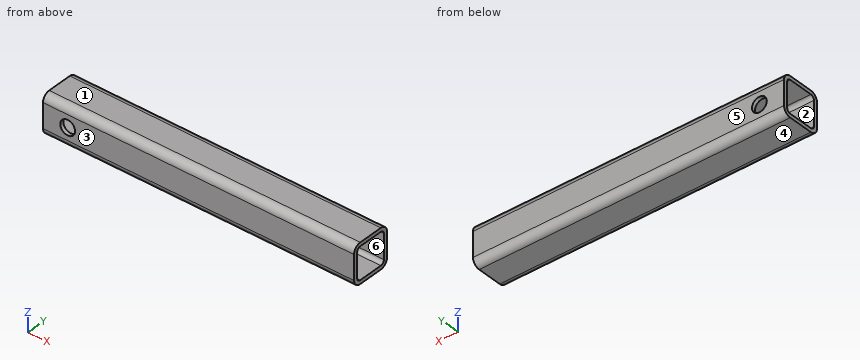
from build123d import *

# Parameters (mm, degrees)
TUBE_SQUARE_TS2X2X0_1875_1_DEPTH = 400
SKETCH12_R                       = 9.525
CUT_EXTRUDE1_DEPTH               = 405.012128531


with BuildPart() as part:
    # Sketch11 → Tube square TS2X2X0.1875(1) (new body)
    with BuildSketch(Plane.YZ):
        with BuildLine():
            Line((-15.875, -25.4), (15.875, -25.4))
            ThreePointArc((15.875, -25.4), (22.610192091, -22.610192091), (25.4, -15.875))
            Line((25.4, -15.875), (25.4, 15.875))
            ThreePointArc((25.4, 15.875), (22.610192091, 22.610192091), (15.875, 25.4))
            Line((15.875, 25.4), (-15.875, 25.4))
            ThreePointArc((-15.875, 25.4), (-22.610192091, 22.610192091), (-25.4, 15.875))
            Line((-25.4, 15.875), (-25.4, -15.875))
            ThreePointArc((-25.4, -15.875), (-22.610192091, -22.610192091), (-15.875, -25.4))
        make_face()
        with BuildLine():
            Line((-15.875, -20.6375), (15.875, -20.6375))
            ThreePointArc((15.875, -20.6375), (19.242596045, -19.242596045), (20.6375, -15.875))
            Line((20.6375, -15.875), (20.6375, 15.875))
            ThreePointArc((20.6375, 15.875), (19.242596045, 19.242596045), (15.875, 20.6375))
            Line((15.875, 20.6375), (-15.875, 20.6375))
            ThreePointArc((-15.875, 20.6375), (-19.242596045, 19.242596045), (-20.6375, 15.875))
            Line((-20.6375, 15.875), (-20.6375, -15.875))
            ThreePointArc((-20.6375, -15.875), (-19.242596045, -19.242596045), (-15.875, -20.6375))
        make_face(mode=Mode.SUBTRACT)
    extrude(amount=TUBE_SQUARE_TS2X2X0_1875_1_DEPTH)

    # Sketch12 → Cut-Extrude1 (cut, through all)
    with BuildSketch(Plane(origin=(0, 25.4, 0), x_dir=(1, 0, 0), z_dir=(0, 1, 0))):
        with Locations(Location((31.75, 0, 0), (0, 0, 270))):
            Circle(SKETCH12_R)
    extrude(amount=-CUT_EXTRUDE1_DEPTH, mode=Mode.SUBTRACT)


solid = part.part
Input: part model. Units: mm. Frame: model coordinates. Face numbers are marked on the shaded views. A direction names the side the tool comes from. Coordinates: 2 decimals unless noted, no trailing zeros. Loops run counter-clockwise (first coordinate to the right, second up) from the corner with the lowest first, then second, coordinate; pieces in that order, holes last. Notation, with made-up numbers: (16.5, 3) -> (31.5, 3) arc R18 cw to (31.5, 11) -> close; hole circle Ø7 at (78, 23.5). An arc over 180 degrees is marked (long way). Write each question's results on one line, items separated by ' | '. Start each with the question number.
Q1. Reachability of the marked faces 5 and 6 from +Z, -Z, +X, -X, +Y, -Y: full face, straight path, thin tool, end or side. Return the list, or none.
Q2. Ray query, line 1 (Z direction, x = 350.5, y = -10.5); line 2 (X direction, y = -24.15, z = 0) (3 decimals). Return the intervals inside material, ascending. Write a range as from..to.
Q3. Pin query (flat end, axial travel): pin 1 (15 mm diameter, centred on x = 31.75, z = 0, fed in from +Y); pin 2 (6 mm diameter, centred on x = 125.5, z = -19.5, fed in from +Y). Return the tip coordinate at first contact, or that it passes through.
Q4. Pull-direction query (Z, two-part tool) for the marked faces 1, 2, 3 and 4; classes: released by +Z, released by -Z, zero draft, split by the parting line, or undercut.
Q5. Section C-C, the plane y = 0.5. Return the cut outline in (x, z).
Q6. Section A-A, the plane z = 0. Return the cut outline in (x, y) (1 decimal).
Found:
1) face 5: +Z, -Z, +X, -X, +Y | face 6: +X, -X
2) line 1: -25.4..-20.64, 20.64..25.4 | line 2: 0..22.225, 41.275..400
3) pin 1: through | pin 2: y = 25.38
4) face 1: released by +Z | face 2: undercut | face 3: zero draft | face 4: released by -Z
5) outline: (0, -25.4) -> (400, -25.4) -> (400, -20.64) -> (0, -20.64) -> close; (0, 20.64) -> (400, 20.64) -> (400, 25.4) -> (0, 25.4) -> close
6) outline: (0, -25.4) -> (22.2, -25.4) -> (22.2, -20.6) -> (0, -20.6) -> close; (0, 20.6) -> (22.2, 20.6) -> (22.2, 25.4) -> (0, 25.4) -> close; (41.3, -25.4) -> (400, -25.4) -> (400, -20.6) -> (41.3, -20.6) -> close; (41.3, 20.6) -> (400, 20.6) -> (400, 25.4) -> (41.3, 25.4) -> close
